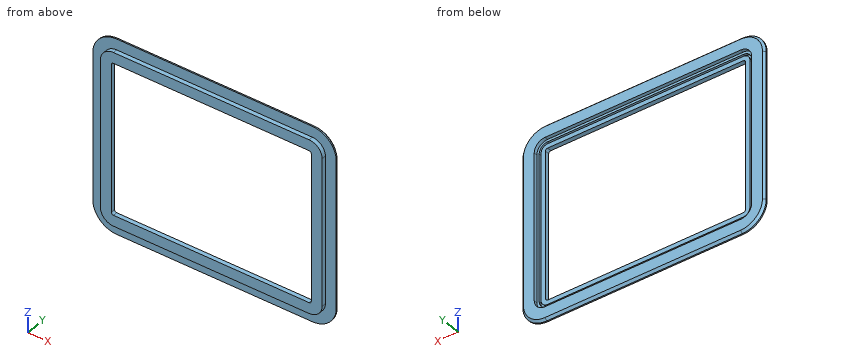
```python
from build123d import *

# Parameters (mm, degrees)
PAD_DEPTH       = 8
PAD001_DEPTH    = 10
POCKET_DEPTH    = 18
POCKET001_DEPTH = 8
POCKET002_DEPTH = 5
CHAMFER_SIZE    = 5


with BuildPart() as part:
    # Sketch → Pad (new body)
    with BuildSketch(Plane.XZ):
        with BuildLine():
            Line((-280, 170), (-280, -170))
            ThreePointArc((-280, -170), (-263.890873, -208.890873), (-225, -225))
            Line((-225, -225), (225, -225))
            ThreePointArc((225, -225), (263.890873, -208.890873), (280, -170))
            Line((280, -170), (280, 170))
            ThreePointArc((280, 170), (263.890873, 208.890873), (225, 225))
            Line((225, 225), (-225, 225))
            ThreePointArc((-225, 225), (-263.890873, 208.890873), (-280, 170))
        make_face()
    extrude(amount=PAD_DEPTH)

    # Sketch001 (on Face10 of Pad) → Pad001 (join)
    with BuildSketch(Plane.XZ.offset(8)):
        with BuildLine():
            Line((-255, 170), (-255, -170))
            ThreePointArc((-255, -170), (-246.213203, -191.213203), (-225, -200))
            Line((-225, -200), (225, -200))
            ThreePointArc((225, -200), (246.213203, -191.213203), (255, -170))
            Line((255, -170), (255, 170))
            ThreePointArc((255, 170), (246.213203, 191.213203), (225, 200))
            Line((225, 200), (-225, 200))
            ThreePointArc((-225, 200), (-246.213203, 191.213203), (-255, 170))
        make_face()
    extrude(amount=PAD001_DEPTH)

    # Sketch002 (on Face4 of Pad001) → Pocket (cut)
    with BuildSketch(Plane(origin=(0, 0, 0), x_dir=(1, 0, 0), z_dir=(0, 1, 0))):
        with BuildLine():
            Line((-230, 170), (-230, -170))
            ThreePointArc((-230, -170), (-228.535534, -173.535534), (-225, -175))
            Line((-225, -175), (225, -175))
            ThreePointArc((225, -175), (228.535534, -173.535534), (230, -170))
            Line((230, -170), (230, 170))
            ThreePointArc((230, 170), (228.535534, 173.535534), (225, 175))
            Line((225, 175), (-225, 175))
            ThreePointArc((-225, 175), (-228.535534, 173.535534), (-230, 170))
        make_face()
    extrude(amount=-POCKET_DEPTH, mode=Mode.SUBTRACT)

    # Sketch003 (on Face4 of Pocket) → Pocket001 (cut)
    with BuildSketch(Plane(origin=(0, 0, 0), x_dir=(1, 0, 0), z_dir=(0, 1, 0))):
        with BuildLine():
            Line((-250, 170), (-250, -170))
            ThreePointArc((-250, -170), (-242.67767, -187.67767), (-225, -195))
            Line((-225, -195), (225, -195))
            ThreePointArc((225, -195), (242.67767, -187.67767), (250, -170))
            Line((250, -170), (250, 170))
            ThreePointArc((250, 170), (242.67767, 187.67767), (225, 195))
            Line((225, 195), (-225, 195))
            ThreePointArc((-225, 195), (-242.67767, 187.67767), (-250, 170))
        make_face()
    extrude(amount=-POCKET001_DEPTH, mode=Mode.SUBTRACT)

    # Sketch004 (on Face27 of Pocket001) → Pocket002 (cut)
    with BuildSketch(Plane(origin=(0, -8, 0), x_dir=(1, 0, 0), z_dir=(0, 1, 0))):
        with BuildLine():
            Line((-244.5, 170), (-244.5, -170))
            ThreePointArc((-244.5, -170), (-238.788582, -183.788582), (-225, -189.5))
            Line((-225, -189.5), (225, -189.5))
            ThreePointArc((225, -189.5), (238.788582, -183.788582), (244.5, -170))
            Line((244.5, -170), (244.5, 170))
            ThreePointArc((244.5, 170), (238.788582, 183.788582), (225, 189.5))
            Line((225, 189.5), (-225, 189.5))
            ThreePointArc((-225, 189.5), (-238.788582, 183.788582), (-244.5, 170))
        make_face()
        with BuildLine():
            Line((-240, 170), (-240, -170))
            ThreePointArc((-240, -170), (-235.606602, -180.606602), (-225, -185))
            Line((-225, -185), (225, -185))
            ThreePointArc((225, -185), (235.606602, -180.606602), (240, -170))
            Line((240, -170), (240, 170))
            ThreePointArc((240, 170), (235.606602, 180.606602), (225, 185))
            Line((225, 185), (-225, 185))
            ThreePointArc((-225, 185), (-235.606602, 180.606602), (-240, 170))
        make_face(mode=Mode.SUBTRACT)
    extrude(amount=-POCKET002_DEPTH, mode=Mode.SUBTRACT)

    # Chamfer
    chamfer_edges = [part.edges().sort_by_distance(p)[0] for p in [
        (0, 0, 225),
        (-263.890873, 0, 208.890873),
        (-280, 0, 0),
        (-263.890873, 0, -208.890873),
        (0, 0, -225),
        (263.890873, 0, -208.890873),
        (280, 0, 0),
        (263.890873, 0, 208.890873),
    ]]
    chamfer(chamfer_edges, length=CHAMFER_SIZE)


solid = part.part
```
Source: CAD feature listing. Evaluate the final solid. Frame: model axes, mm. Coordinates: 2 decimals unless noted, no trailing zeros. Order: outer loops, then holes, each group sorted by start corner. A loop starts at its lowest first (then second) coordinate and runs counter-clockwise, first axis right, second up. Notation, with made-up numbers: (68.5, -15.5) - (127.5, -15.5) arc R7 ccw to (127.5, -10.5) - close; hole circle Ø8 at (-19, 30.25). An arc over 180 degrees is marked (long way). One line per item, written item: value.
1) Cut plane A-A on x = 27. Output: boundary loops of the cut face in (y, z), plus the area to 3 significant figures.
Computed values:
outline: (-18, -200) - (-8, -200) - (-8, -225) - (-5, -225) - (0, -220) - (0, -195) - (-8, -195) - (-8, -189.5) - (-13, -189.5) - (-13, -185) - (-8, -185) - (-8, -175) - (-18, -175) - close; (-18, 175) - (-8, 175) - (-8, 185) - (-13, 185) - (-13, 189.5) - (-8, 189.5) - (-8, 195) - (0, 195) - (0, 220) - (-5, 225) - (-8, 225) - (-8, 200) - (-18, 200) - close
area: 910 mm^2
2) Ray query, line 1 (Z direction, x = 167, y = -10.75); line 2 (X direction, y = -12.5, z = 167); line 3 (Z direction, x = -1, y = -16.5). Return the intervals inside material, ascending. Write a range as [from, to].
Computed values:
line 1: z = [-200, -189.5], [-185, -175], [175, 185], [189.5, 200]
line 2: x = [-255, -244.5], [-240, -230], [230, 240], [244.5, 255]
line 3: z = [-200, -175], [175, 200]
3) Contact query for flat-ended pins moving along their axis: pin 1 (5 mm diameter, centred on y = -14.5, z = -65.5, fed in from -X); pin 2 (4 mm diameter, centred on x = -112, y = -11, fed in from -Z); pin 3 (1.5 mm diameter, centred on y = -9.5, z = 72, fed in from +X). Output: stop coordinate, or through.
Computed values:
pin 1: stops at x = -255
pin 2: stops at z = -200
pin 3: stops at x = 255
4) Cut plane B-B on z = -139. Output: boundary loops of the cut face in (x, y), plus the area to 3 significant figures.
Computed values:
outline: (-280, -8) - (-255, -8) - (-255, -18) - (-230, -18) - (-230, -8) - (-240, -8) - (-240, -13) - (-244.5, -13) - (-244.5, -8) - (-250, -8) - (-250, 0) - (-275, 0) - (-280, -5) - close; (230, -18) - (255, -18) - (255, -8) - (280, -8) - (280, -5) - (275, 0) - (250, 0) - (250, -8) - (244.5, -8) - (244.5, -13) - (240, -13) - (240, -8) - (230, -8) - close
area: 910 mm^2
